```python
from build123d import *

# Parameters (mm, degrees)
SKETCH4_W           = 50
SKETCH4_H           = 32
BOSS_EXTRUDE1_DEPTH = 25
SKETCH5_R           = 2
CUT_EXTRUDE1_DEPTH  = 5
SKETCH2_R           = 2.5
SKETCH2_R_2         = 2
BOSS_EXTRUDE2_DEPTH = 1
SKETCH7_R           = 4
SKETCH7_R_2         = 1.6
BOSS_EXTRUDE3_DEPTH = 1
FILLET1_R           = 2.5
SKETCH8_R           = 12.5
BOSS_EXTRUDE4_DEPTH = 45
SKETCH10_R          = 4
BOSS_EXTRUDE5_DEPTH = 2
SKETCH11_R          = 1
BOSS_EXTRUDE6_DEPTH = 1
FILLET2_R           = 0.5


with BuildPart() as part:
    # Sketch4 → Boss-Extrude1 (new body)
    with BuildSketch(Plane(origin=(83.969208633, 0, 0), x_dir=(0, 0, -1), z_dir=(1, 0, 0))):
        with Locations((-28, 7.3)):
            Rectangle(SKETCH4_W, SKETCH4_H)
    extrude(amount=BOSS_EXTRUDE1_DEPTH)

    # Sketch5 → Cut-Extrude1 (cut)
    with BuildSketch(Plane.ZY.offset(-83.969208633)):
        with Locations((8, 18.8)):
            Circle(SKETCH5_R)
        with Locations((48, 18.8)):
            Circle(SKETCH5_R)
        with Locations((48, -4.2)):
            Circle(SKETCH5_R)
        with Locations((8, -4.2)):
            Circle(SKETCH5_R)
    extrude(amount=-CUT_EXTRUDE1_DEPTH, mode=Mode.SUBTRACT)

    # Sketch2 → Boss-Extrude2 (add)
    with BuildSketch(Plane(origin=(108.969208633, 0, 0), x_dir=(0, 0, -1), z_dir=(1, 0, 0))):
        with Locations((-48, 18.8)):
            Circle(SKETCH2_R)
        with Locations((-48, 18.8)):
            Circle(SKETCH2_R_2, mode=Mode.SUBTRACT)
        with Locations((-8, 18.8)):
            Circle(SKETCH2_R)
        with Locations((-8, 18.8)):
            Circle(SKETCH2_R_2, mode=Mode.SUBTRACT)
        with Locations((-8, -4.2)):
            Circle(SKETCH2_R)
        with Locations((-8, -4.2)):
            Circle(SKETCH2_R_2, mode=Mode.SUBTRACT)
        with Locations((-48, -4.2)):
            Circle(SKETCH2_R)
        with Locations((-48, -4.2)):
            Circle(SKETCH2_R_2, mode=Mode.SUBTRACT)
    extrude(amount=BOSS_EXTRUDE2_DEPTH)

    # Sketch7 → Boss-Extrude3 (add)
    with BuildSketch(Plane(origin=(108.969208633, 0, 0), x_dir=(0, 0, -1), z_dir=(1, 0, 0))):
        with Locations((-28, 7.3)):
            Circle(SKETCH7_R)
        with Locations((-24, 11.3)):
            Circle(SKETCH7_R_2)
        with Locations((-24, 3.3)):
            Circle(SKETCH7_R_2)
    extrude(amount=BOSS_EXTRUDE3_DEPTH)

    # Fillet1
    fillet1_edges = [part.edges().sort_by_distance(p)[0] for p in [
        (96.469208633, 23.3, 53),
        (96.469208633, 23.3, 3),
        (96.469208633, -8.7, 3),
        (96.469208633, -8.7, 53),
    ]]
    fillet(fillet1_edges, radius=FILLET1_R)

    # Sketch8 → Boss-Extrude4 (add)
    with BuildSketch(Plane.XY.offset(53)):
        with Locations((98.969208633, 7.3)):
            Circle(SKETCH8_R)
    extrude(amount=BOSS_EXTRUDE4_DEPTH)

    # Sketch10 → Boss-Extrude5 (add)
    with BuildSketch(Plane.XY.offset(98)):
        with Locations((98.969208633, 7.3)):
            Circle(SKETCH10_R)
    extrude(amount=BOSS_EXTRUDE5_DEPTH)

    # Sketch11 → Boss-Extrude6 (add)
    with BuildSketch(Plane.XY.offset(100)):
        with Locations((98.969208633, 7.3)):
            Circle(SKETCH11_R)
    extrude(amount=BOSS_EXTRUDE6_DEPTH)

    # Fillet2
    fillet2_edges = [part.edges().sort_by_distance(p)[0] for p in [
        (94.969208633, 7.3, 98),
        (94.969208633, 7.3, 100),
    ]]
    fillet(fillet2_edges, radius=FILLET2_R)


solid = part.part
```
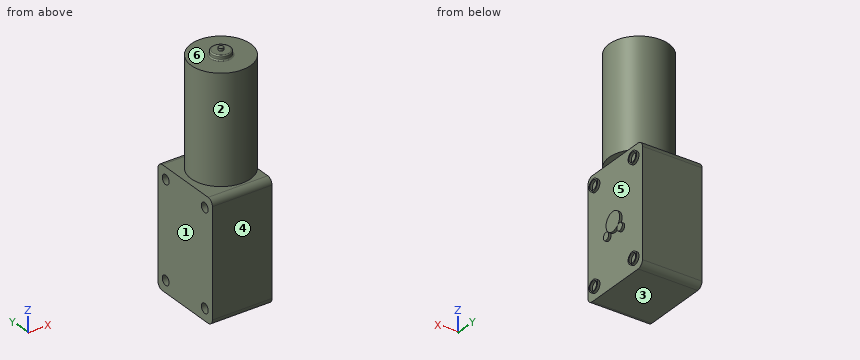
The listing builds one solid part. Answer for the finished solid, in the listing's coordinates (mm). Face numbers are marked on the shaded views. A direction names the side the tool comes from. Give positions to 0.01 mm unless a question says otherwise; leave off trailing zeros. Order: outer loops, then holes, each group sorted by start corner. A loop starts at its lowest first (then second) coordinate and runs counter-clockwise, first axis right, second up.
1) Determine the mould class of the marked faces 3, 4, 5 and 6 for opening direction Z: pulls with the +Z half, pulls with the -Z half, needs draft (parallel to the pull), parting line crosses it, or undercut.
Reported:
face 3: pulls with the -Z half
face 4: needs draft
face 5: undercut
face 6: pulls with the +Z half
2) Given P1, Ø1.5, axis at y = 12.5, z = 27.5, coming from the +X side; P2, Ø2, axis at x = 99.5, y = 10.5, coming from the +Z side; P3, Ø5.5, axis at y = 18.5, z = 47.5, coming from the +X side, each flat-ended and moving along its own axis, determine where each tip first touches the part or whether it passes through.
Reported:
P1: stops at x = 108.97
P2: stops at z = 100
P3: stops at x = 109.97
3) Find section A-A on z = 48. Write down the section's boundary in (x, y).
Reported:
outline: (83.97, -8.7) - (108.97, -8.7) - (108.97, -6.7) - (109.97, -6.7) - (109.97, -6.2) - (108.97, -6.2) - (108.97, -2.2) - (109.97, -2.2) - (109.97, -1.7) - (108.97, -1.7) - (108.97, 16.3) - (109.97, 16.3) - (109.97, 16.8) - (108.97, 16.8) - (108.97, 20.8) - (109.97, 20.8) - (109.97, 21.3) - (108.97, 21.3) - (108.97, 23.3) - (83.97, 23.3) - (83.97, 20.8) - (88.97, 20.8) - (88.97, 16.8) - (83.97, 16.8) - (83.97, -2.2) - (88.97, -2.2) - (88.97, -6.2) - (83.97, -6.2) - close
4) Find section C-C on x = 107.5. Write down the section's boundary in (y, z).
Reported:
outline: (-8.7, 5.5) arc R2.5 ccw to (-6.2, 3) - (20.8, 3) arc R2.5 ccw to (23.3, 5.5) - (23.3, 50.5) arc R2.5 ccw to (20.8, 53) - (16.44, 53) - (16.44, 98) - (-1.84, 98) - (-1.84, 53) - (-6.2, 53) arc R2.5 ccw to (-8.7, 50.5) - close
5) Consider line 1 along Y through (x, z) = (109.6, 8); line 2 along Y through (x, z) = (85.4, 48); line 3 along X through (y, z) = (20, 21). Determine where each line is inside the solid, lowest interval first.
Reported:
line 1: y = -6.7 to -6.2, -2.2 to -1.7, 16.3 to 16.8, 20.8 to 21.3
line 2: y = -8.7 to -6.2, -2.2 to 16.8, 20.8 to 23.3
line 3: x = 83.97 to 108.97
6) For the marked faces 1 and 2, determine the directions among +Z, -Z, +X, -X, +Y, -Y from which every point of the face is accessible in a straight line to the end or side of a thin tool.
Reported:
face 1: +Z, -Z, -X, +Y, -Y
face 2: +Z
7) Find section D-D on z = 28. Write down the section's boundary in (x, y), then the cut area to 3 significant figures.
Reported:
outline: (83.97, -8.7) - (108.97, -8.7) - (108.97, 3.3) - (109.97, 3.3) - (109.97, 11.3) - (108.97, 11.3) - (108.97, 23.3) - (83.97, 23.3) - close
area: 808 mm2
8) Find section B-B on y = 7.3. Write down the section's boundary in (x, z), then the cut area to 3 significant figures.
Reported:
outline: (83.97, 3) - (108.97, 3) - (108.97, 24) - (109.97, 24) - (109.97, 32) - (108.97, 32) - (108.97, 53) - (111.47, 53) - (111.47, 98) - (103.47, 98) arc R0.5 cw to (102.97, 98.5) - (102.97, 99.5) arc R0.5 ccw to (102.47, 100) - (99.97, 100) - (99.97, 101) - (97.97, 101) - (97.97, 100) - (95.47, 100) arc R0.5 ccw to (94.97, 99.5) - (94.97, 98.5) arc R0.5 cw to (94.47, 98) - (86.47, 98) - (86.47, 53) - (83.97, 53) - close
area: 2,400 mm2
